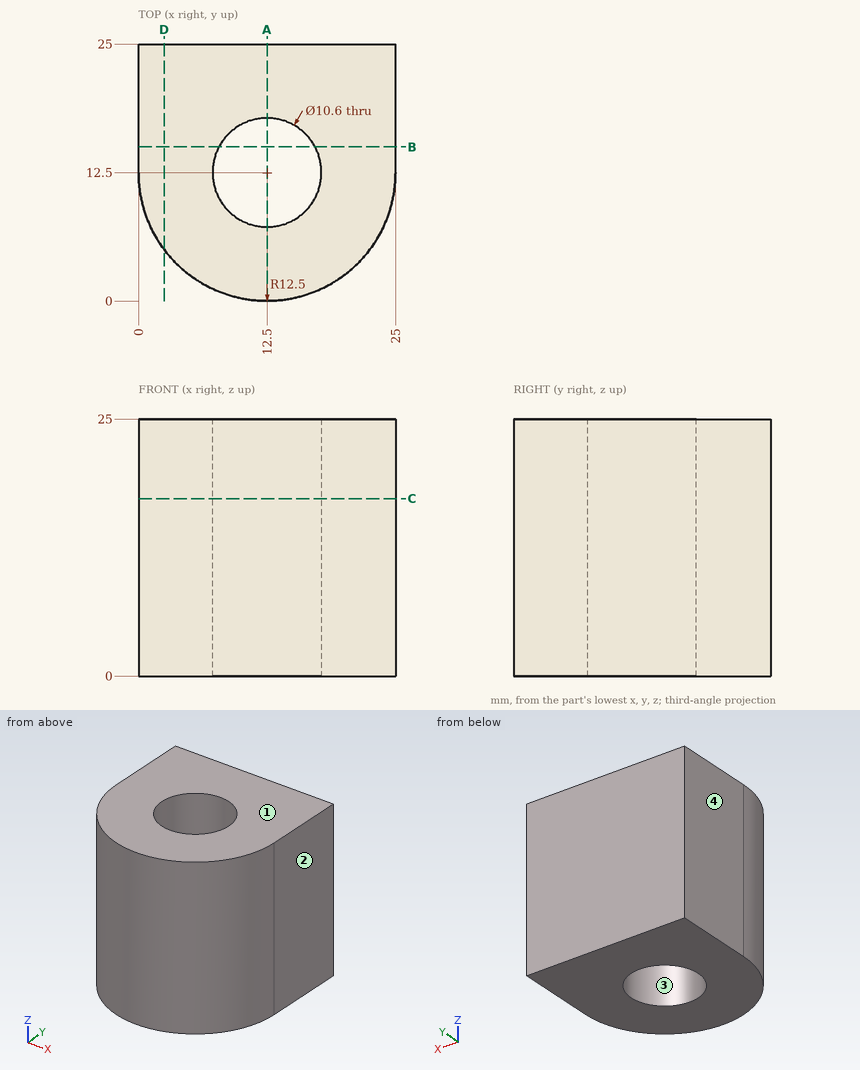
The drawing under review shows one solid part. Ordinate dimensions are in mm from its lowest x, y, z. Round coordinates to 2 decimals unless told otherwise and drop trailing zeros. Loops run counter-clockwise (first coordinate to the right, second up) from the corner with the lowest first, then second, coordinate; pieces in that order, holes last. Notation, with made-up numbers: (60, 1) - (97, 1) arc R20 cw to (97, 7) - close; hole circle Ø6 at (58.5, 85). An arc over 180 degrees is marked (long way). One line per item, written item: value. Start each with the question number.
1) Consider section D-D on x = 2.5. Give the boundary of the cut face in (y, z).
2) Consider section C-C on z = 17.25. Give the boundary of the cut face in (x, y).
3) Consider section B-B on y = 15. Give the boundary of the cut face in (x, z), then the cut area to 3 significant figures.
4) To check wall thickness, follow L1, parallel to Y at x = 12.5, z = 16.75; L2, parallel to Y at x = 9.5, z = 22.5; L3, parallel to X at y = 16.25, z = 5.25. State the ranges of each line that lie inside material, in increasing order. Write a range as from..to.
5) Consider section A-A on x = 12.5. Give the boundary of the cut face in (y, z).
6) Draft analysis for pull direction X (two halves, no side actions). For the marked faces 1, 2, 3 and 4, state which applies: +X half, -X half, draft (parallel to the pull), parting line (faces both ways), or undercut.
7) Insertion check: pin 1 Ø4 at (y, z) = (6.5, 21.5) entering from -X; pin 2 Ø5 at (x, z) = (21, 17.5) entering from -Y; pin 3 Ø3 at (y, z) = (6.5, 5.5) entering from +X; pin 4 Ø8.5 at (x, y) = (12.5, 12.5) entering from +Z. Each pin has a flat end and moves straight along its axis. Give the tip position at first contact, or say it passes through.
Reported:
1. outline: (5, 0) - (25, 0) - (25, 25) - (5, 25) - close
2. outline: (0, 12.5) arc R12.5 ccw to (25, 12.5) - (25, 25) - (0, 25) - close; hole circle Ø10.6 at (12.5, 12.5)
3. outline: (0, 0) - (7.83, 0) - (7.83, 25) - (0, 25) - close; (17.17, 0) - (25, 0) - (25, 25) - (17.17, 25) - close
3. area: 391 mm^2
4. L1: y = 0..7.2, 17.8..25
4. L2: y = 0.37..8.13, 16.87..25
4. L3: x = 0..8.75, 16.25..25
5. outline: (0, 0) - (7.2, 0) - (7.2, 25) - (0, 25) - close; (17.8, 0) - (25, 0) - (25, 25) - (17.8, 25) - close
6. face 1: draft
6. face 2: +X half
6. face 3: undercut
6. face 4: -X half
7. pin 1: stops at x = 0.66
7. pin 2: stops at y = 1.53
7. pin 3: stops at x = 24.16
7. pin 4: passes through
